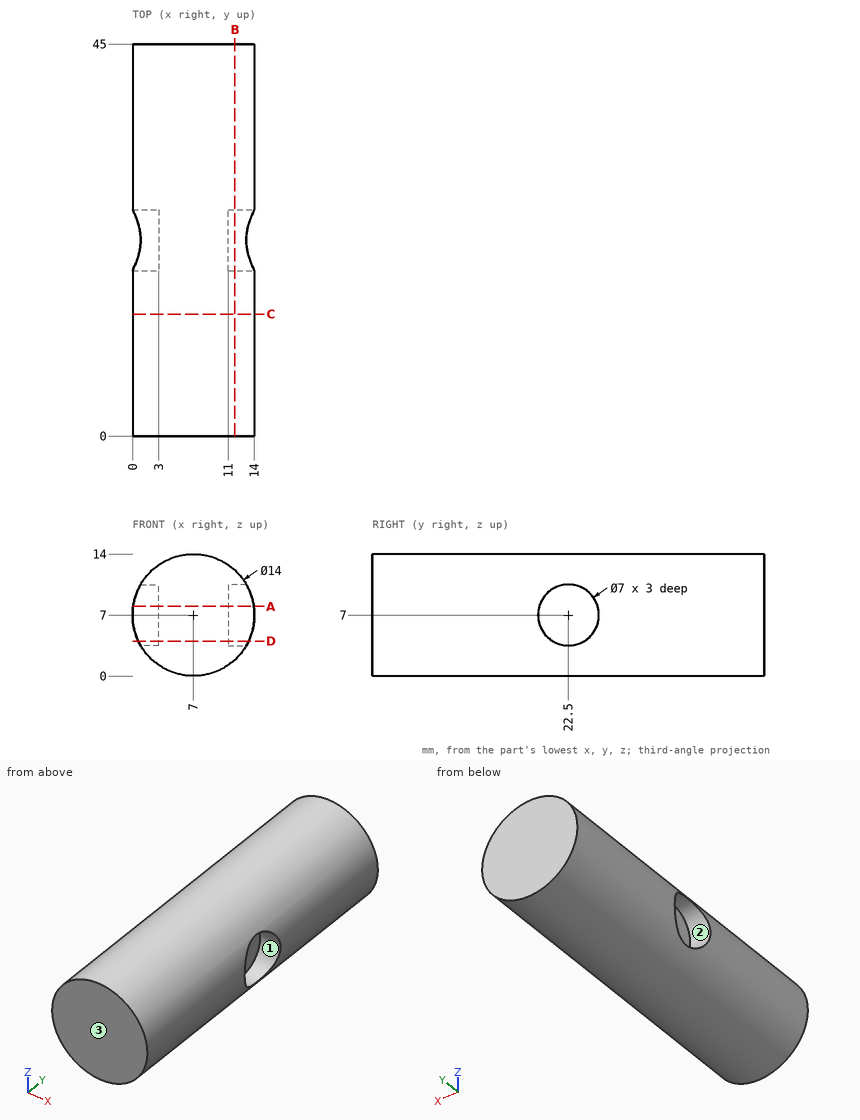
Here's the drawing with two shaded views (mm, measured from the low corner). I have some questions. A direction names the side the tool comes from. Give positions to 0.01 mm unless a question says otherwise; leave off trailing zeros. Write each loop counter-clockwise with the first axis right and the second up, starting at its lowest first coordinate (ties: lowest second). Pieces come first, ordered by that corner, then holes. Notation, with made-up numbers: (22.5, 42) - (75.5, 42) arc R33 cw to (75.5, 78) - close; hole circle Ø5 at (53.5, 82). An arc over 180 degrees is marked (long way). One line per item, written item: value. Start each with the question number.
Item 1: Please list where these lines run through material, in increasing order: line 1 (Y direction, x = 13.1, z = 7); line 2 (X direction, y = 39, z = 12.75); line 3 (Y direction, x = 11.5, z = 9.75). Write a range as from..to.
Item 2: Imagine slicing it at C-C, the plane y = 14. List the corners of the cut face in (x, z) for me, and give its area (3 significant figures).
Item 3: Which directions (+Z, -Z, +X, -X, +Y, -Y) give clear straight access to the entire face, cutting with the end or side of a thin tool? Please do the marked faces 1, 2 and 3.
Item 4: Imagine slicing it at D-D, the plane z = 4. List the corners of the cut face in (x, y) for me.
Item 5: Imagine slicing it at B-B, the plane x = 11.75. List the corners of the cut face in (y, z) for me.
Item 6: I'm going to push flat-ended pins straight in: pin 1 (1.5 mm diameter, centred on x = 3, y = 20.5, fed in from -Z); pin 2 (3.5 mm diameter, centred on y = 24, z = 6.5, fed in from +X); pin 3 (8 mm diameter, centred on x = 2.5, y = 35, fed in from +Z). Where does each tip first touch, or does it pass through?
Item 7: Imagine slicing it at A-A, the plane z = 8. List the corners of the cut face in (x, y) for me.
Geometry says:
1. line 1: 0..19, 26..45
1. line 2: 3.01..10.99
1. line 3: 0..20.33, 24.67..45
2. outline: circle Ø14 at (7, 7)
2. area: 154 mm^2
3. face 1: +X
3. face 2: -X
3. face 3: +Z, -Z, +X, -X, -Y
4. outline: (0.68, 0) - (13.32, 0) - (13.32, 20.7) - (11, 20.7) - (11, 24.3) - (13.32, 24.3) - (13.32, 45) - (0.68, 45) - (0.68, 24.3) - (3, 24.3) - (3, 20.7) - (0.68, 20.7) - close
5. outline: (0, 1.86) - (45, 1.86) - (45, 12.14) - (0, 12.14) - close; hole circle Ø7 at (22.5, 7)
6. pin 1: z = 0.8
6. pin 2: x = 11
6. pin 3: z = 13.98
7. outline: (0.07, 0) - (13.93, 0) - (13.93, 19.15) - (11, 19.15) - (11, 25.85) - (13.93, 25.85) - (13.93, 45) - (0.07, 45) - (0.07, 25.85) - (3, 25.85) - (3, 19.15) - (0.07, 19.15) - close
